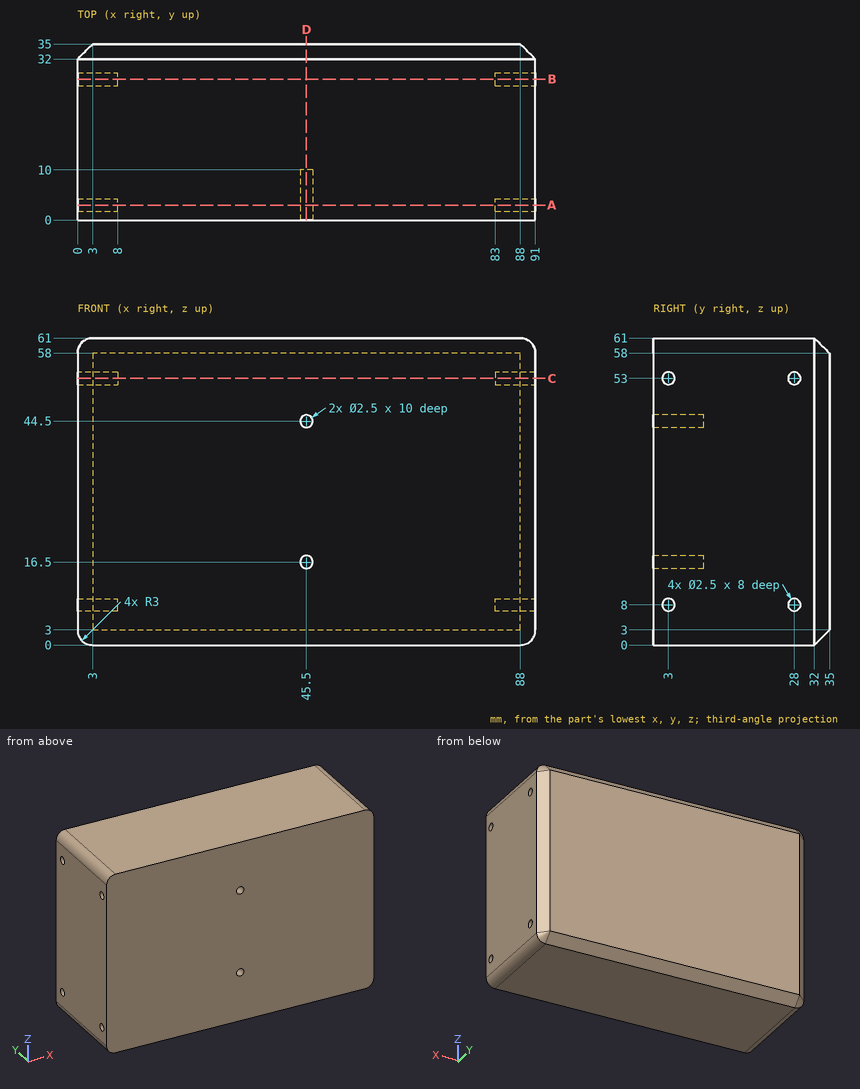
Print and shaded views of the part. All mm, measured from the part's lowest x, y and z. Round coordinates to 2 decimals unless told otherwise and drop trailing zeros. Write each loop counter-clockwise with the first axis right and the second up, starting at its lowest first coordinate (ties: lowest second). Pieces come first, ordered by that corner, then holes.
(1) Slice it at D-D, the plane x = 45.5. Write the cut outline in (y, z).
(2) Drop flat-ended pins along their axis: P1, Ø1.5, axis at y = 3, z = 53, coming from the +X side; P2, Ø1.2, axis at x = 45.5, z = 16.5, coming from the -Y side; P3, Ø2, axis at y = 3, z = 8, coming from the -X side. Give the stop position or say it passes through.
(3) Slice it at C-C, the plane z = 53. Write the cut outline in (x, y), and give its area (3 significant figures).
(4) Probe line 1 along Y through (x, z) = (85, 8); line 2 along X through (y, z) = (2.5, 7); line 3 along X through (y, z) = (2, 16). List the from-to ranges inside material, lowest first.
(5) Slice it at B-B, the plane y = 28. Write the cut outline in (x, z).
(6) Slice it at A-A, the plane y = 3. Write the cut outline in (x, z), and give its area (3 significant figures).
From the geometry:
1. outline: (0, 0) - (32, 0) - (35, 3) - (35, 58) - (32, 61) - (0, 61) - (0, 45.75) - (10, 45.75) - (10, 43.25) - (0, 43.25) - (0, 17.75) - (10, 17.75) - (10, 15.25) - (0, 15.25) - close
2. P1: stops at x = 83
2. P2: stops at y = 10
2. P3: stops at x = 8
3. outline: (0, 0) - (91, 0) - (91, 1.75) - (83, 1.75) - (83, 4.25) - (91, 4.25) - (91, 26.75) - (83, 26.75) - (83, 29.25) - (91, 29.25) - (91, 32) - (88, 35) - (3, 35) - (0, 32) - (0, 29.25) - (8, 29.25) - (8, 26.75) - (0, 26.75) - (0, 4.25) - (8, 4.25) - (8, 1.75) - (0, 1.75) - close
3. area: 3,100 mm2
4. line 1: y = 0 to 1.75, 4.25 to 26.75, 29.25 to 35
4. line 2: x = 8 to 83
4. line 3: x = 0 to 44.35, 46.65 to 91
5. outline: (0, 3) arc R3 ccw to (3, 0) - (88, 0) arc R3 ccw to (91, 3) - (91, 6.75) - (83, 6.75) - (83, 9.25) - (91, 9.25) - (91, 51.75) - (83, 51.75) - (83, 54.25) - (91, 54.25) - (91, 58) arc R3 ccw to (88, 61) - (3, 61) arc R3 ccw to (0, 58) - (0, 54.25) - (8, 54.25) - (8, 51.75) - (0, 51.75) - (0, 9.25) - (8, 9.25) - (8, 6.75) - (0, 6.75) - close
6. outline: (0, 3) arc R3 ccw to (3, 0) - (88, 0) arc R3 ccw to (91, 3) - (91, 6.75) - (83, 6.75) - (83, 9.25) - (91, 9.25) - (91, 51.75) - (83, 51.75) - (83, 54.25) - (91, 54.25) - (91, 58) arc R3 ccw to (88, 61) - (3, 61) arc R3 ccw to (0, 58) - (0, 54.25) - (8, 54.25) - (8, 51.75) - (0, 51.75) - (0, 9.25) - (8, 9.25) - (8, 6.75) - (0, 6.75) - close; hole circle Ø2.5 at (45.5, 16.5); hole circle Ø2.5 at (45.5, 44.5)
6. area: 5,450 mm2
